from build123d import *

# Parameters (mm, degrees)
SKETCH2_W               = 80
SKETCH2_H               = 120
SKETCH2_W_2             = 64
SKETCH2_H_2             = 104
BOSS_EXTRUDE1_DEPTH     = 2200
FILLET4_R               = 15
SKETCH4_R               = 15
BOSS_EXTRUDE2_DEPTH     = 16
FILLET1_R               = 30
FILLET2_R               = 150
FILLET1_OF_MIRROR1_R    = 30
FILLET2_OF_MIRROR1_R    = 150
SKETCH5_R               = 15
BOSS_EXTRUDE3_DEPTH     = 16
FILLET3_R               = 150
SKETCH9_R               = 15
BOSS_EXTRUDE4_DEPTH     = 8
FILLET5_R               = 30
FILLET3_OF_MIRROR5_R    = 150
FILLET5_OF_MIRROR5_R    = 30
CUT_EXTRUDE1_DEPTH      = 17
CUT_EXTRUDE1_DEPTH_BACK = 97


with BuildPart() as part:
    # Sketch2 → Boss-Extrude1 (new body)
    with BuildSketch(Plane(origin=(0, 0, 0), x_dir=(0, 0, -1), z_dir=(1, 0, 0))):
        with Locations((0, 80)):
            Rectangle(SKETCH2_W, SKETCH2_H)
        with Locations((0, 80)):
            Rectangle(SKETCH2_W_2, SKETCH2_H_2, mode=Mode.SUBTRACT)
    extrude(amount=BOSS_EXTRUDE1_DEPTH)

    # Fillet4
    fillet4_edges = [part.edges().sort_by_distance(p)[0] for p in [
        (1100, 132, 32),
        (1100, 28, 32),
        (1100, 28, -32),
        (1100, 132, -32),
        (1100, 20, -40),
        (1100, 20, 40),
        (1100, 140, 40),
        (1100, 140, -40),
    ]]
    fillet(fillet4_edges, radius=FILLET4_R)

    # Sketch4 → Boss-Extrude2 (add)
    with BuildSketch(Plane.XY.offset(40)):
        with BuildLine():
            Line((663.616754147, 140), (0, 140))
            Line((0, 140), (-46.702488681, 17.857142857))
            ThreePointArc((-46.702488681, 17.857142857), (-35.438939598, -35.271540371), (17.635818001, -46.786514333))
            Line((17.635818001, -46.786514333), (141.756963012, 0))
            Line((141.756963012, 0), (163.853984354, -79.985767518))
            ThreePointArc((163.853984354, -79.985767518), (193.903117134, -107.0010543), (231.031250542, -91.054963543))
            Line((231.031250542, -91.054963543), (306.382973978, 20))
            Line((306.382973978, 20), (663.616754147, 20))
            ThreePointArc((663.616754147, 20), (723.616754147, 80), (663.616754147, 140))
        make_face()
        Circle(SKETCH4_R, mode=Mode.SUBTRACT)
        with Locations((200, -70)):
            Circle(SKETCH4_R, mode=Mode.SUBTRACT)
    boss_extrude2 = extrude(amount=BOSS_EXTRUDE2_DEPTH)

    # Fillet1
    fillet1_edges = [part.edges().sort_by_distance(p)[0] for p in [
        (141.756963012, 0, 48),
    ]]
    fillet(fillet1_edges, radius=FILLET1_R)

    # Fillet2
    fillet2_edges = [part.edges().sort_by_distance(p)[0] for p in [
        (306.382973978, 20, 48),
    ]]
    fillet(fillet2_edges, radius=FILLET2_R)

    # Mirror1: Boss-Extrude2 across plane
    add(boss_extrude2.mirror(Plane(origin=(0, 0, 0), x_dir=(1, 0, 0), z_dir=(0, 0, -1))))

    # Fillet1 of Mirror1
    fillet1_of_mirror1_edges = [part.edges().sort_by_distance(p)[0] for p in [
        (141.756963012, 0, -48),
    ]]
    fillet(fillet1_of_mirror1_edges, radius=FILLET1_OF_MIRROR1_R)

    # Fillet2 of Mirror1
    fillet2_of_mirror1_edges = [part.edges().sort_by_distance(p)[0] for p in [
        (306.382973978, 20, -48),
    ]]
    fillet(fillet2_of_mirror1_edges, radius=FILLET2_OF_MIRROR1_R)



with BuildPart() as body_2:
    # Sketch5 → Boss-Extrude3 (new body)
    with BuildSketch(Plane.XY.offset(40)):
        with BuildLine():
            ThreePointArc((2156.472909481, 20.031536396), (2270.867590896, 59.441328796), (2330, 165))
            ThreePointArc((2330, 165), (2315.741185035, 190.538502182), (2286.518993754, 191.800419224))
            Line((2286.518993754, 191.800419224), (2216.86153125, 156.761687956))
            Line((2216.86153125, 156.761687956), (2143.638230406, 138.15116888))
            ThreePointArc((2143.638230406, 138.15116888), (2098.769091881, 73.518650853), (2156.472909481, 20.031536396))
        make_face()
        with Locations((2300, 165)):
            Circle(SKETCH5_R, mode=Mode.SUBTRACT)
    boss_extrude3 = extrude(amount=BOSS_EXTRUDE3_DEPTH)

    # Fillet3
    fillet3_edges = [body_2.edges().sort_by_distance(p)[0] for p in [
        (2216.86153125, 156.761687956, 48),
    ]]
    fillet(fillet3_edges, radius=FILLET3_R)


with BuildPart() as part_1:
    add(part.part)

    add(body_2.part)  # Boss-Extrude4 merges body 2
    # Sketch9 → Boss-Extrude4 (add)
    with BuildSketch(Plane.XY.offset(40)):
        with BuildLine():
            Line((1610, 140), (2157.550798688, 140))
            Line((2157.550798688, 140), (2157.550798688, 20))
            Line((2157.550798688, 20), (1524.006966774, 18.707022476))
            ThreePointArc((1524.006966774, 18.707022476), (1469.944566534, 51.119453365), (1473.059803349, 114.07661416))
            Line((1473.059803349, 114.07661416), (1555.063784392, 236.678883391))
            ThreePointArc((1555.063784392, 236.678883391), (1588.715317888, 248.706153245), (1610, 220))
            Line((1610, 220), (1610, 140))
        make_face()
        with Locations((1580, 220)):
            Circle(SKETCH9_R, mode=Mode.SUBTRACT)
    boss_extrude4 = extrude(amount=BOSS_EXTRUDE4_DEPTH)

    # Fillet5
    fillet5_edges = [part_1.edges().sort_by_distance(p)[0] for p in [
        (1610, 140, 44),
    ]]
    fillet(fillet5_edges, radius=FILLET5_R)

    # Mirror5: Boss-Extrude3, Boss-Extrude4 across plane
    add(boss_extrude3.mirror(Plane(origin=(0, 0, 0), x_dir=(1, 0, 0), z_dir=(0, 0, -1))))
    add(boss_extrude4.mirror(Plane(origin=(0, 0, 0), x_dir=(1, 0, 0), z_dir=(0, 0, -1))))

    # Fillet3 of Mirror5
    fillet3_of_mirror5_edges = [part_1.edges().sort_by_distance(p)[0] for p in [
        (2216.86153125, 156.761687956, -48),
    ]]
    fillet(fillet3_of_mirror5_edges, radius=FILLET3_OF_MIRROR5_R)

    # Fillet5 of Mirror5
    fillet5_of_mirror5_edges = [part_1.edges().sort_by_distance(p)[0] for p in [
        (1610, 140, -44),
    ]]
    fillet(fillet5_of_mirror5_edges, radius=FILLET5_OF_MIRROR5_R)

    # Sketch6 → Cut-Extrude1 (cut, two sides)
    with BuildSketch(Plane.XY.offset(40)) as cut_extrude1_sk:
        with BuildLine():
            Line((1827.553025368, 100), (2002.553025368, 100))
            ThreePointArc((2002.553025368, 100), (2022.553025368, 80), (2002.553025368, 60))
            Line((2002.553025368, 60), (1827.553025368, 60))
            ThreePointArc((1827.553025368, 60), (1807.553025368, 80), (1827.553025368, 100))
        make_face()
    extrude(amount=CUT_EXTRUDE1_DEPTH, mode=Mode.SUBTRACT)
    extrude(cut_extrude1_sk.sketch, amount=-CUT_EXTRUDE1_DEPTH_BACK, mode=Mode.SUBTRACT)


solid = part_1.part
Model file for the job. Use its own axes, mm. A direction names the side the tool comes from. Give positions to 0.01 mm unless a question says otherwise; leave off trailing zeros. Loops run counter-clockwise (first coordinate to the right, second up) from the corner with the lowest first, then second, coordinate; pieces in that order, holes last.
Item 1: Drop flat-ended pins along their axis: P1, Ø9, axis at x = 1903, z = -43.5, coming from the +Y side; P2, Ø1.5, axis at x = 585, z = 7.5, coming from the -Y side; P3, Ø1.5, axis at y = 25, z = 19, coming from the +X side. Give the stop position or say it passes through.
Check values:
P1: stops at y = 140
P2: stops at y = 20
P3: stops at x = 2200
Item 2: Slice it at A-A (x = 1054.5). Write the cut outline in (y, z).
Check values:
outline: (20, -25) arc R15 ccw to (35, -40) - (125, -40) arc R15 ccw to (140, -25) - (140, 25) arc R15 ccw to (125, 40) - (35, 40) arc R15 ccw to (20, 25) - close; hole (28, -17) arc R15 ccw to (43, -32) - (117, -32) arc R15 ccw to (132, -17) - (132, 17) arc R15 ccw to (117, 32) - (43, 32) arc R15 ccw to (28, 17) - close
Item 3: Drill centre lines: line 1 along Z through (x, y) = (92.5, 81); line 2 along Y through (x, z) = (394, 2.5); line 3 along Y through (x, z) = (1580, 43.25). Where is each one in solid material? Low to high.
Check values:
line 1: z = -56 to -32, 32 to 56
line 2: y = 20 to 28, 132 to 140
line 3: y = 18.82 to 205, 235 to 250
Item 4: Which spindle directions (+Z, -Z, +X, -X, +Y, -Y) get a long thin tool onto all of the face, cutting with end or side? Do faces 5 (the face through (2098.65, 74.71, 51.94)), 6 (the face through (2200, 81, 36)), 7 (the face through (213, 26, 40)). Say none if no direction does.
Check values:
face 5: +Z
face 6: +X, +Y, -Y
face 7: none
Item 5: Mould opens along Y. For faces 1 (the face through (1085, 79, 32)), 2 (the face through (723.602, 78.681, -47.888)), 3 (the face through (1513.49, 174.52, -43.94)), 4 (the face through (0, 81, 36)) say: +Y half, -Y half, draft (parallel to the pull), parting line (faces both ways), or undercut.
Check values:
face 1: undercut
face 2: parting line
face 3: +Y half
face 4: draft
